Build history of the part. All positions in model axes, mm. A direction names the side the tool comes from. Round coordinates to 2 decimals unless told otherwise and drop trailing zeros. Write each loop counter-clockwise with the first axis right and the second up, starting at its lowest first coordinate (ties: lowest second). Pieces come first, ordered by that corner, then holes. Notation, with made-up numbers: (-35.75, -15.5) -> (20.25, -15.5) arc R13 cw to (20.25, -9.5) -> close; hole circle Ø2 at (24, 45). An arc over 180 degrees is marked (long way). One line per question, with ' | ' between items.
from build123d import *

# Parameters (mm, degrees)
SKETCH1_W           = 60
SKETCH1_H           = 40
BOSS_EXTRUDE1_DEPTH = 40
SKETCH5_W           = 36
SKETCH5_H           = 38
CUT_EXTRUDE3_DEPTH  = 83.462112512
SKETCH6_R           = 4
CUT_EXTRUDE4_DEPTH  = 83.462112512


with BuildPart() as part:
    # Sketch1 → Boss-Extrude1 (new body)
    with BuildSketch(Plane(origin=(0, 0, 0), x_dir=(1, 0, 0), z_dir=(0, 1, 0))):
        with Locations((30, 20)):
            Rectangle(SKETCH1_W, SKETCH1_H)
    extrude(amount=BOSS_EXTRUDE1_DEPTH)

    # Sketch5 → Cut-Extrude3 (cut, through all)
    with BuildSketch(Plane(origin=(60, 0, 0), x_dir=(0, 0, -1), z_dir=(1, 0, 0))):
        with Locations((20, 21)):
            Rectangle(SKETCH5_W, SKETCH5_H)
    extrude(amount=-CUT_EXTRUDE3_DEPTH, mode=Mode.SUBTRACT)

    # Sketch6 → Cut-Extrude4 (cut, through all)
    with BuildSketch(Plane.XY):
        Polygon((10, 15), (0, 0), (0, 40), (60, 40), align=None)
        with Locations((25, 7)):
            Circle(SKETCH6_R)
        with Locations((50, 25)):
            Circle(SKETCH6_R)
    extrude(amount=-CUT_EXTRUDE4_DEPTH, mode=Mode.SUBTRACT)


solid = part.part
(1) Slice it at B-B (y = 25). Write the cut outline in (x, z), then the cut area to 3 significant figures.
Calculated:
outline: (30, -40) -> (46, -40) -> (46, -38) -> (30, -38) -> close; (30, -2) -> (46, -2) -> (46, 0) -> (30, 0) -> close; (54, -40) -> (60, -40) -> (60, -38) -> (54, -38) -> close; (54, -2) -> (60, -2) -> (60, 0) -> (54, 0) -> close | area: 88.0 mm2
(2) 3-axis set-ups, long thin cutter, end or side, ignore diameter. For faces 1 (the cylindrical face through (21, 7, -1)), 2 (the flat face through (38, 17, -2)): which of +Z, -Z, +X, -X, +Y, -Y reach the whole face in a straight line?
Calculated:
face 1: +Z, -Z | face 2: +X, -X, +Y
(3) Slice it at D-D (x = 11). Write the cut outline in (y, z), then the cut area to 3 significant figures.
Calculated:
outline: (0, -40) -> (15.5, -40) -> (15.5, -38) -> (2, -38) -> (2, -2) -> (15.5, -2) -> (15.5, 0) -> (0, 0) -> close | area: 134 mm2
(4) Mould opens along Z. For faces 3 (the flat face through (36, 15, -40)), 4 (the flat face through (31, 2, -20)), 5 (the flat face through (0.949, 1.424, -21.388)) say: pulls with the +Z half, pulls with the -Z half, needs draft (parallel to the pull), parting line crosses it, or undercut.
Calculated:
face 3: pulls with the -Z half | face 4: undercut | face 5: needs draft
(5) Drop flat-ended pins along their axis: pin 1 (6.5 mm diameter, centred on x = 25, y = 7, fed in from +Z); pin 2 (11 mm diameter, centred on x = 40, z = -26.5, fed in from +Y). Give the stop position or say it passes through.
Calculated:
pin 1: through | pin 2: y = 2
(6) Slice it at A-A (x = 25). Write the cut outline in (y, z).
Calculated:
outline: (0, -40) -> (3, -40) -> (3, -38) -> (2, -38) -> (2, -2) -> (3, -2) -> (3, 0) -> (0, 0) -> close; (11, -40) -> (22.5, -40) -> (22.5, -38) -> (11, -38) -> close; (11, -2) -> (22.5, -2) -> (22.5, 0) -> (11, 0) -> close
(7) Slice it at C-C (y = 16). Write the cut outline in (x, z).
Calculated:
outline: (12, -40) -> (60, -40) -> (60, -38) -> (12, -38) -> close; (12, -2) -> (60, -2) -> (60, 0) -> (12, 0) -> close
(8) Wall check: line 1 (Y direction, x = 41.5, z = -11.5); line 2 (Z direction, x = 13, y = 8); line 3 (Y direction, x = 50, z = -38.45). Give the ranges that are in metal, low to high. Write a range as from..to.
Calculated:
line 1: 0..2 | line 2: -40..-38, -2..0 | line 3: 0..21, 29..35
